Here's how the part is built. I have some questions about the finished solid (model axes, mm). A direction names the side the tool comes from. Give positions to 0.01 mm unless a question says otherwise; leave off trailing zeros. Loops run counter-clockwise (first coordinate to the right, second up) from the corner with the lowest first, then second, coordinate; pieces in that order, holes last.
Q1. Suppose I cut it at A-A (y = 0). List the corners of the cut face in (x, z) for me, and give its area (3 significant figures).
Q2. Suppose I cut it at C-C (z = 68). List the corners of the cut face in (x, y) for me, and give its area (3 significant figures).
Q3. I'm going to push a flat-ended pin straight in: P1, Ø3, axis at x = 3, z = 52.5, coming from the +Y side. Where does the tip first touch, or does it pass through?
Q4. For faces 1 (the face through (0, -1, 20)), 2 (the face through (15, 0, 49)), 3 (the face through (0, 0, 0)), 4 (the face through (29, 0, 80)), which set-ups out of +Z, -Z, +X, -X, +Y, -Y let a thin tool reach every point of the face, with its end or its side?
Q5. I need wall thicknesses on probe 1 along Z at (x, y) = (17.5, -0.1); probe 2 along X at (y, z) = (-0.1, 66.5); probe 3 along X at (y, z) = (0.15, 35.5). Which ranges of each line are inside material? Lowest first, please.
Q6. Suppose I cut it at B-B (x = 17.5). List the corners of the cut face in (y, z) for me.
```python
from build123d import *

# Parameters (mm, degrees)
SKETCH_1_R = 1


with BuildPart() as part:
    # ｽｲｰﾌﾟ1: sweep along a path in ｽｹｯﾁ2
    with BuildLine(Plane(origin=(0, 0, 0), x_dir=(1, 0, 0), z_dir=(0, 1, 0))) as sweep_1_path:
        Line((0, 0), (0, -40))
        ThreePointArc((0, -40), (2.928932188, -47.071067812), (10, -50))
        Line((10, -50), (20, -50))
        ThreePointArc((20, -50), (27.071067812, -52.928932188), (30, -60))
        Line((30, -60), (30, -100))
    # ｽｹｯﾁ1 → ｽｲｰﾌﾟ1 (sweep)
    with BuildSketch(Plane.XY):
        Circle(SKETCH_1_R)
    sweep(path=sweep_1_path.line)


solid = part.part
```
Solutions:
1. outline: (-1, 0) - (1, 0) - (1, 40) arc R9 cw to (10, 49) - (20, 49) arc R11 ccw to (31, 60) - (31, 100) - (29, 100) - (29, 60) arc R9 cw to (20, 51) - (10, 51) arc R11 ccw to (-1, 40) - close
1. area: 243 mm2
2. outline: circle Ø2 at (30, 0)
2. area: 3.14 mm2
3. P1: passes through
4. face 1: -Z
4. face 2: none
4. face 3: -Z, +X, -X, +Y, -Y
4. face 4: +Z
5. probe 1: z = 49.01 to 50.99
5. probe 2: x = 29.01 to 30.99
5. probe 3: x = -0.99 to 0.99
6. outline: circle Ø2 at (0, 50)
